Check sheet for the modelled part. Datum: model origin and axes. Units: mm. A direction names the side the tool comes from. Coordinates: 2 decimals unless noted, no trailing zeros. Loops run counter-clockwise (first coordinate to the right, second up) from the corner with the lowest first, then second, coordinate; pieces in that order, holes last. Notation, with made-up numbers: (-34.75, 36) -> (-21.75, 36) arc R26 cw to (-21.75, 53) -> close; hole circle Ø1 at (66.5, 70). An arc over 180 degrees is marked (long way). Use CSV: the item, a comma, the result in double quotes. Start each with the question number.
1. Set-up check for faces 4 (the face through (57, -25.5, -25)), 5 (the face through (8, 13.2, -2)), 6 (the face through (-12, 7, 0)), 7 (the face through (22.4, 1.87, 12.54)), 8 (the face through (-17, -4, -1)): record each of +Z, -Z, +X, -X, +Y, -Y from which the full face is reachable in a straight line by a thin tool's end or side.
2. Sectioned sample at B-B, the plane x = 83. Record the cut outline in (y, z), and give its area (3 significant figures).
3. Sectioned sample at A-A, the plane y = 5.5. Record the cut outline in (x, z), and give its area (3 significant figures).
4. Thickness scan on L1, parallel to Z at x = 95.5, y = 25; L2, parallel to Z at x = 7, y = -9; L3, parallel to X at y = -1.5, z = -32.5. Record the ranges inside material, lowest first.
5. Sectioned sample at C-C, the plane z = -31. Record the cut outline in (x, y), and give its area (3 significant figures).
6. Gauge pin test, flat ends, axial feed: pin 1 (3 mm diameter, centred on y = -2, z = -41, fed in from -X); pin 2 (10 mm diameter, centred on x = 88.5, z = 4.5, fed in from -Y); pin 3 (0.6 mm diameter, centred on x = -1, z = -1, fed in from +Y); pin 4 (8 mm diameter, centred on x = -9, z = -13.5, fed in from +Y). Record the tip position at first contact, or that the pin passes through.
7. Sectioned sample at D-D, the plane y = -20. Record the cut outline in (x, z), and give its area (3 significant figures).
8. Release check for a two-part mould opening along X. For faces 1 (the face through (-3.4, -1.7, 4)), 2 (the face through (12, 0, -44)), 3 (the face through (10, -20, -18.5)) record: pulls with the +X half, pulls with the -X half, needs draft (parallel to the pull), parting line crosses it, or undercut.
Autodesk Inventor part; units mm, degrees
ref_plane "P3_XY" through (-12.5, 0, 0) normal (1, 0, 0) x (0, 0, -1)
ref_plane "P3_YZ" through (-12.5, 0, 0) normal (0, 0, -1) x (0, 1, 0)
ref_plane "P3_ZX" through (-12.5, 0, 0) normal (0, 1, 0) x (1, 0, 0)
sketch "Sketch_2" plane through (0, 0, 0) normal (0, 1, 0) x (-1, 0, 0)
  line L0 (0, -26) -> (0, 15)
  line L1 (0, 15) -> (-91.3632, 15)
  line L2 (-91.3632, 15) -> (-92.533, -18.5)
  line L3 (-92.533, -18.5) -> (-102, -18.5)
  line L4 (-102, -18.5) -> (-102, -61)
  line L5 (-102, -61) -> (-12, -61)
  line L6 (-12, -61) -> (-12, -26)
  line L7 (-12, -26) -> (0, -26)
extrude "Extrusion1" add sketch "Sketch_2" along normal mid plane 54
sketch "Sketch_3" plane through (0, 0, 0) normal (1, 0, 0) x (0, 1, 0)
  line L0 (-30, 19) -> (-30, -26)
  line L1 (-30, -26) -> (-27, -26)
  line L2 (-27, -26) -> (-25.75, 8.0894)
  line L3 (-25.75, 8.0894) -> (-25.75, 12.7365)
  arc A0 (-5.46, 15.3565) -> (-25.75, 12.7365) centre (-5.46, -64.5185) ccw
  line L4 (-5.46, 15.3565) -> (5.46, 15.3565)
  arc A1 (25.75, 12.7365) -> (5.46, 15.3565) centre (5.46, -64.5185) ccw
  line L5 (25.75, 12.7365) -> (25.75, 8.0894)
  line L6 (25.75, 8.0894) -> (27, -26)
  line L7 (27, -26) -> (30, -26)
  line L8 (30, -26) -> (30, 19)
  line L9 (30, 19) -> (-30, 19)
extrude "Extrusion2" cut sketch "Sketch_3" along normal blind 102
sketch "Sketch_4" plane through (0, 0, 0) normal (1, 0, 0) x (0, 1, 0)
  line L0 (22.5, -26) -> (22.5, -26.2)
  line L1 (22.5, -26.2) -> (27, -26.2)
  line L2 (27, -26.2) -> (27, -26)
  line L3 (27, -26) -> (22.5, -26)
extrude "Extrusion3" cut sketch "Sketch_4" along normal blind 102
sketch "Sketch_5" plane through (0, 0, 0) normal (1, 0, 0) x (0, 1, 0)
  line L0 (-22.5, -26) -> (-27, -26)
  line L1 (-27, -26) -> (-27, -26.2)
  line L2 (-27, -26.2) -> (-22.5, -26.2)
  line L3 (-22.5, -26.2) -> (-22.5, -26)
extrude "Extrusion4" cut sketch "Sketch_5" along normal blind 102
sketch "Sketch_6" plane through (0, 27, 0) normal (0, 1, 0) x (1, 0, 0)
  line L0 (34, 23.2) -> (80, 23.2)
  line L1 (80, 23.2) -> (80, 26)
  line L2 (80, 26) -> (34, 26)
  line L3 (34, 26) -> (34, 23.2)
extrude "Extrusion5" cut sketch "Sketch_6" against normal blind 1.5
sketch "Sketch_7" plane through (0, -27, 0) normal (0, 1, 0) x (1, 0, 0)
  line L0 (34, 23.2) -> (80, 23.2)
  line L1 (80, 23.2) -> (80, 26)
  line L2 (80, 26) -> (34, 26)
  line L3 (34, 26) -> (34, 23.2)
extrude "Extrusion6" cut sketch "Sketch_7" along normal blind 1.5
sketch "Sketch_8" plane through (0, 0, -18.5) normal (0, 0, 1) x (1, 0, 0)
  line L0 (-10, -30) -> (20, -30)
  line L1 (20, -30) -> (20, -16.8)
  arc A0 (20, -16.8) -> (16.4, -13.2) centre (16.4, -16.8) ccw
  line L2 (16.4, -13.2) -> (-5, -13.2)
  line L3 (-5, -13.2) -> (-5, 13.2)
  line L4 (-5, 13.2) -> (16.4, 13.2)
  arc A1 (16.4, 13.2) -> (20, 16.8) centre (16.4, 16.8) ccw
  line L5 (20, 16.8) -> (20, 30)
  line L6 (20, 30) -> (-10, 30)
  line L7 (-10, 30) -> (-10, -30)
extrude "Extrusion7" cut sketch "Sketch_8" along normal blind 38.5
sketch "Sketch_9" plane through (0, 0, 0) normal (1, 0, 0) x (0, 1, 0)
  arc A0 (-2.5617, 4) -> (-4, 2.5617) centre (0, 0) ccw
  line L0 (-4, 2.5617) -> (-4, -2.5617)
  arc A1 (-4, -2.5617) -> (-2.5617, -4) centre (0, 0) ccw
  line L1 (-2.5617, -4) -> (2.5617, -4)
  arc A2 (2.5617, -4) -> (4, -2.5617) centre (0, 0) ccw
  line L2 (4, -2.5617) -> (4, 2.5617)
  arc A3 (4, 2.5617) -> (2.5617, 4) centre (0, 0) ccw
  line L3 (2.5617, 4) -> (-2.5617, 4)
extrude "Extrusion8" add sketch "Sketch_9" against normal blind 12.5
sketch "Sketch_10" plane through (-2, 0, 0) normal (1, 0, 0) x (0, 0, -1)
  line L0 (-7, -5.02) -> (-5.02, -7)
  line L1 (-5.02, -7) -> (7, -7)
  line L2 (7, -7) -> (7, 7)
  line L3 (7, 7) -> (-7, 7)
  line L4 (-7, 7) -> (-7, -5.02)
  line L5 (-4.2, -1.3009) -> (-4.2, -1.7397)
  line L6 (-4.2, -1.7397) -> (-1.7397, -4.2)
  line L7 (-1.7397, -4.2) -> (-1.3009, -4.2)
  line L8 (-1.3009, -4.2) -> (-1.1009, -4)
  line L9 (-1.1009, -4) -> (2.5617, -4)
  arc A0 (2.5617, -4) -> (4, -2.5617) centre (0, 0) ccw
  line L10 (4, -2.5617) -> (4, 2.5617)
  arc A1 (4, 2.5617) -> (2.5617, 4) centre (0, 0) ccw
  line L11 (2.5617, 4) -> (-2.5617, 4)
  arc A2 (-2.5617, 4) -> (-4, 2.5617) centre (0, 0) ccw
  line L12 (-4, 2.5617) -> (-4, -1.1009)
  line L13 (-4, -1.1009) -> (-4.2, -1.3009)
extrude "Extrusion9" add sketch "Sketch_10" against normal blind 20
sketch "Sketch_11" plane through (-22, 0, 0) normal (1, 0, 0) x (0, 0, -1)
  line L0 (-2.195, -7) -> (0, -11.7072)
  line L1 (0, -11.7072) -> (2.195, -7)
  line L2 (2.195, -7) -> (-2.195, -7)
extrude "Extrusion10" add sketch "Sketch_11" along normal blind 3
sketch "Sketch_1" plane through (0, 0, 10) normal (0, 0, 1) x (1, 0, 0)
  line L0 (16.804, 0.696) -> (16.804, -0.696)
  arc A0 (16.804, -0.696) -> (17.804, -1.696) centre (17.804, -0.696) ccw
  line L1 (17.804, -1.696) -> (21.196, -1.696)
  arc A1 (21.196, -1.696) -> (22.196, -0.696) centre (21.196, -0.696) ccw
  line L2 (22.196, -0.696) -> (22.196, 0.696)
  arc A2 (22.196, 0.696) -> (21.196, 1.696) centre (21.196, 0.696) ccw
  line L3 (21.196, 1.696) -> (17.804, 1.696)
  arc A3 (17.804, 1.696) -> (16.804, 0.696) centre (17.804, 0.696) ccw
extrude "Extrusion11" cut sketch "Sketch_1" along normal blind 8 draft 15
ref_plane "P3_XY" through (-12.5, 0, 0) normal (1, 0, 0) x (0, 0, -1)
ref_plane "P3_YZ" through (-12.5, 0, 0) normal (0, 0, -1) x (0, 1, 0)
ref_plane "P3_ZX" through (-12.5, 0, 0) normal (0, 1, 0) x (1, 0, 0)
properties part number "100031_P3"
Completed:
1,face 4,"-Y"
1,face 5,"+Z, -X, +Y"
1,face 6,"+Z, -Z, -X, +Y"
1,face 7,"+Z"
1,face 8,"-X"
2,outline,"(-27, -61) -> (27, -61) -> (27, -26.2) -> (22.5, -26.2) -> (22.5, -26) -> (27, -26) -> (25.75, 8.09) -> (25.75, 12.74) arc R79.87 ccw to (13, 15) -> (-13, 15) arc R79.88 ccw to (-25.75, 12.74) -> (-25.75, 8.09) -> (-27, -26) -> (-22.5, -26) -> (-22.5, -26.2) -> (-27, -26.2) -> close"
2,area,"4,020 mm²"
3,outline,"(-22, -7) -> (-2, -7) -> (-2, 7) -> (-22, 7) -> close; (0, -26) -> (12, -26) -> (12, -61) -> (102, -61) -> (102, -18.5) -> (92.53, -18.5) -> (91.36, 15) -> (0, 15) -> close"
3,area,"7,280 mm²"
4,L1,"-61 to -26.2, -26 to -18.5"
4,L2,"-26 to 15"
4,L3,"12 to 102"
5,outline,"(12, -27) -> (102, -27) -> (102, 27) -> (12, 27) -> close"
5,area,"4,860 mm²"
6,pin 1,"x = 12"
6,pin 2,"y = -26.06"
6,pin 3,"y = 4"
6,pin 4,"through"
7,outline,"(0, -26) -> (12, -26) -> (12, -61) -> (102, -61) -> (102, -18.5) -> (92.53, -18.5) -> (91.4, 14.02) -> (20, 14.02) -> (20, -18.5) -> (0, -18.5) -> close"
7,area,"6,260 mm²"
8,face 1,"undercut"
8,face 2,"pulls with the -X half"
8,face 3,"needs draft"
